from build123d import *

# Parameters (mm, degrees)
BOSS_EXTRUDE1_DEPTH = 3
SKETCH2_R           = 0.95
CUT_EXTRUDE1_DEPTH  = 3


with BuildPart() as part:
    # Model → Boss-Extrude1 (new body)
    with BuildSketch(Plane.XY):
        Polygon((3.28114864, -0.553591744), (3.683973872, -0.606311596), (3.904576525, -0.692596416), (4.46233576, -1.16335455), (4.354682595, -1.543555198), (3.63291812, -1.652020067), (3.399826682, -1.609842083), (3.029159111, -1.443549864), (2.651791815, -2.076361715), (2.974290661, -2.323428597), (3.122197977, -2.508452992), (3.369848791, -3.195022478), (3.08652147, -3.47046279), (2.407220835, -3.20351854), (2.226450258, -3.050441439), (1.98859116, -2.721092688), (1.345375685, -3.080440385), (1.501144473, -3.455651839), (1.536726867, -3.689840852), (1.407911756, -4.40825247), (1.024820816, -4.505118707), (0.570002205, -3.934287195), (0.489986205, -3.711334195), (0.448670194, -3.307180093), (-0.288044489, -3.296769041), (-0.340764213, -3.69959429), (-0.427049372, -3.92019681), (-0.897807506, -4.477956045), (-1.278008415, -4.370303805), (-1.386473285, -3.64853933), (-1.344295476, -3.415447861), (-1.178003257, -3.04478029), (-1.810815108, -2.667412994), (-2.05788199, -2.98991184), (-2.242905897, -3.137819766), (-2.929475702, -3.385469696), (-3.204916014, -3.102142375), (-2.937971765, -2.422841739), (-2.784894663, -2.242071162), (-2.455545912, -2.004212065), (-2.814890389, -1.360994791), (-3.190106124, -1.516753266), (-3.424295137, -1.55233566), (-4.142706929, -1.423521518), (-4.239572929, -1.040430518), (-3.668740929, -0.585612518), (-3.445787929, -0.505596518), (-3.041633929, -0.464279518), (-3.031233208, 0.272435311), (-3.434058457, 0.325155035), (-3.65466111, 0.411439855), (-4.212419929, 0.882198482), (-4.104767689, 1.262399392), (-3.383003067, 1.370863283), (-3.149911423, 1.328686443), (-2.779244225, 1.162393392), (-2.401877369, 1.795205505), (-2.724376698, 2.042271757), (-2.872284136, 2.227296053), (-3.119934385, 2.913865744), (-2.836607064, 3.189306056), (-2.157306429, 2.922361806), (-1.976536269, 2.769284211), (-1.738676514, 2.439935935), (-1.09545924, 2.799280412), (-1.251217361, 3.174496294), (-1.286799755, 3.408685307), (-1.157985613, 4.127097098), (-0.774894613, 4.223963098), (-0.320076613, 3.653131098), (-0.240060613, 3.430178098), (-0.198743613, 3.026024098), (0.53797107, 3.015613046), (0.590690923, 3.418438278), (0.676975742, 3.639040931), (1.147733877, 4.196800166), (1.527934524, 4.089147), (1.636398415, 3.367382378), (1.5942214, 3.134290766), (1.427928349, 2.763623568), (2.060740462, 2.386256712), (2.307806714, 2.708756041), (2.492831498, 2.856662868), (3.179400869, 3.104314002), (3.454841181, 2.820986681), (3.187896932, 2.141686046), (3.03481983, 1.960915469), (2.705471079, 1.723056371), (3.064815556, 1.079839097), (3.440031438, 1.235597218), (3.674220451, 1.271179612), (4.392632069, 1.142364502), (4.489498306, 0.759273562), (3.918666794, 0.30445495), (3.695713794, 0.22443895), (3.291559693, 0.18312294), align=None)
    extrude(amount=BOSS_EXTRUDE1_DEPTH)

    # Sketch2 → Cut-Extrude1 (cut)
    with BuildSketch(Plane.XY.offset(3)):
        Circle(SKETCH2_R)
    extrude(amount=-CUT_EXTRUDE1_DEPTH, mode=Mode.SUBTRACT)


solid = part.part
The model under review builds one solid part; all positions refer to its coordinate system, in mm. Coordinates: 2 decimals unless noted, no trailing zeros. Loops run counter-clockwise (first coordinate to the right, second up) from the corner with the lowest first, then second, coordinate; pieces in that order, holes last. Notation, with made-up numbers: M 46,41 L 103,41 A25 cw 103,74 Z; hole C -9,81 d5. An arc over 180 degrees is marked long. Put each result on its own line as item: value. Start each with the question number.
Q1. The part is to be moulded in two halves that separate along X. For faces 1 (the flat face through (1.2, -0.1, 3)), 2 (the cylindrical face through (-0.95, 0.04, 1.52)), say which applies: +X half, -X half, draft (parallel to the pull), parting line (faces both ways), or undercut.
Q2. Add section A-A (x = 0). Write out the cut boundary in (y, z).
Q3. Wall thickness on line 1 (X direction, y = 2.5, z = 1.2); line 2 (X direction, y = 2, z = 2.2); line 3 (Y direction, x = 0, z = 1.55): over which ranges is each line inside the solid? List them lowest first.
Q4. Clearance check with flat-ended pins moving along their axes: pin 1 (2 mm diameter, centred on x = 0, y = 0, fed in from -Z); pin 2 (1.5 mm diameter, centred on x = -3.5, z = 1, fed in from +Y). State where each tip first meets the part, or that it passes through.
Q5. Add section B-B (y = 0). Write out the cut boundary in (x, z), and give its area (3 significant figures).
Answers:
1. face 1: draft
1. face 2: undercut
2. outline: M -3.3,0 L -0.95,0 L -0.95,3 L -3.3,3 Z; M 0.95,0 L 3.02,0 L 3.02,3 L 0.95,3 Z
3. line 1: x = -2.97 to -1.78, -1.63 to 1.87, 2.15 to 3.33
3. line 2: x = -2.67 to 3.07
3. line 3: y = -3.3 to -0.95, 0.95 to 3.02
4. pin 1: stops at z = 0
4. pin 2: stops at y = 3.19
5. outline: M -3.04,0 L -0.95,0 L -0.95,3 L -3.04,3 Z; M 0.95,0 L 3.29,0 L 3.29,3 L 0.95,3 Z
5. area: 13.3 mm^2
